Here's how the part is built. I have some questions about the finished solid (model axes, mm). A direction names the side the tool comes from. Round coordinates to 2 decimals unless told otherwise and drop trailing zeros. Loops run counter-clockwise (first coordinate to the right, second up) from the corner with the lowest first, then second, coordinate; pieces in that order, holes last. Notation, with made-up numbers: M 18,18 L 43,18 A24 cw 43,33 Z; hole C 13,54.5 d5. An arc over 180 degrees is marked long. Answer as a JSON object with one key per item and string values.
from build123d import *

# Parameters (mm, degrees)
F2_DEPTH  = 38.1
F3_W      = 25.4
F3_H      = 31.75
F4_DEPTH  = 25.4
F5_DEPTH  = 12.7
F7_D      = 12.7
F9_DEPTH  = 12.7
F10_DEPTH = 123
F11_R     = 5.08
F13_D     = 6.35
F15_D     = 6.35
F17_D     = 6.35


# Not quite as in the source:
# - an extrude ends at something that could not be found from the text; its depth is read off the source's solid


with BuildPart() as f2:
    # F0 (on Front) → F2 (new body)
    with BuildSketch(Plane.XZ):
        Polygon((-15.0914756011, 53.4695235106), (-53.1914756011, 53.4695235106), (-53.1914756011, 15.3695235106), (10.3085243989, 15.3695235106), (10.3085243989, 21.7195235106), (-15.0914756011, 21.7195235106), align=None)
    extrude(amount=F2_DEPTH)

    # F3 (on face) → F4 (cut)
    with BuildSketch(Plane.YZ.offset(-15.0914756011)):
        with Locations((-25.4, 37.5945235106)):
            Rectangle(F3_W, F3_H)
    extrude(amount=-F4_DEPTH, mode=Mode.SUBTRACT)

    # F5 (cut): a face of the model
    f5_faces = [f2.faces().sort_by_distance(p)[0] for p in [
        (-40.4914756011, -25.4, 37.5945235106),
    ]]
    extrude(f5_faces, amount=-F5_DEPTH, mode=Mode.SUBTRACT)

    # F7 (through all)
    with Locations(Plane.XZ.offset(12.7)):
        with Locations((-40.4914756011, 40.7695235106)):
            Hole(F7_D / 2)

    # F8 (on face) → F9 (cut)
    with BuildSketch(Plane.XZ.offset(12.7)):
        with BuildLine():
            ThreePointArc((-53.1914756011, 40.0317125094), (-40.0621213537, 52.2842661721), (-27.8065160195, 39.1577604642))
            Line((-27.8065160195, 39.1577604642), (-27.8065160195, 34.4195235106))
            ThreePointArc((-27.8065160195, 34.4195235106), (-24.0770508865, 25.4383560684), (-15.0914756011, 21.7195235106))
            Line((-15.0914756011, 21.7195235106), (-15.0914756011, 53.4695235106))
            Line((-15.0914756011, 53.4695235106), (-53.1914756011, 53.4695235106))
            Line((-53.1914756011, 53.4695235106), (-53.1914756011, 40.0317125094))
        make_face()
    extrude(amount=-F9_DEPTH, mode=Mode.SUBTRACT)

    # F1 (on face) → F10 (cut, through all)
    with BuildSketch(Plane.XZ):
        Polygon((-15.0914756011, 21.7195235106), (-15.0914756011, 53.4695235106), (-53.1914756011, 53.4695235106), (-53.1914756011, 15.3695235106), (10.3085243989, 15.3695235106), (10.3085243989, 21.7195235106), align=None)
    extrude(amount=-F10_DEPTH, mode=Mode.SUBTRACT)

    # F11
    f11_edges = [f2.edges().sort_by_distance(p)[0] for p in [
        (-53.191476, -38.1, 18.544524),
        (10.308524, -38.1, 18.544524),
    ]]
    fillet(f11_edges, radius=F11_R)

    # F13 (through all)
    with Locations(Plane.XY.offset(21.7195235106)):
        with Locations((-43.6664756011, -28.575)):
            Hole(F13_D / 2)

    # F15 (through all)
    with Locations(Plane.XY.offset(21.7195235106)):
        with Locations((0.7835243989, -9.525)):
            Hole(F15_D / 2)

    # F17 (through all)
    with Locations(Plane.XY.offset(21.7195235106)):
        with Locations((0.7835243989, -28.575)):
            Hole(F17_D / 2)


solid = f2.part
Item 1: On a 3-axis mill with a long thin cutter (end or side, diameter ignored), from which of +Z, -Z, +X, -X, +Y, -Y can I reach the whole of each face in a straight line? I mean faces 1 (the face through (-27.807, -6, 37)), 2 (the face through (8.86, -36.57, 18.59)). Say none if no direction works.
Resolved:
{"face 1": "+Z, +X, +Y, -Y", "face 2": "+Z, -Z, +X, -Y"}
Item 2: I want a section at B-B, the plane x = -36. Please give me the cut outline in (y, z).
Resolved:
{"outline": "M -38.1,15.37 L 0,15.37 L 0,36.28 L -12.7,36.28 L -12.7,21.72 L -38.1,21.72 Z; M -12.7,45.26 L 0,45.26 L 0,51.47 L -12.7,51.47 Z"}
Item 3: I want a section at C-C, the plane y = -30. Please give me the cut outline in (x, z), then the cut area to 3 significant figures.
Resolved:
{"outline": "M -53.19,15.37 L -46.5,15.37 L -46.5,21.72 L -53.19,21.72 Z; M -40.83,15.37 L -2.05,15.37 L -2.05,21.72 L -40.83,21.72 Z; M 3.62,15.37 L 10.31,15.37 L 10.31,21.72 L 3.62,21.72 Z", "area": "331 mm²"}
Item 4: I want a section at D-D, the plane x = 3. Please give me the cut outline in (y, z), then the cut area to 3 significant figures.
Resolved:
{"outline": "M -38.1,15.37 L -30.85,15.37 L -30.85,21.72 L -38.1,21.72 Z; M -26.3,15.37 L -11.8,15.37 L -11.8,21.72 L -26.3,21.72 Z; M -7.25,15.37 L 0,15.37 L 0,21.72 L -7.25,21.72 Z", "area": "184 mm²"}
Item 5: I'm going to push flat-ended pins straight in: pin 1 Ø6 at (x, y) = (-21, -8.5) entering from +Z; pin 2 Ø1 at (y, z) = (-9, 31) entering from +X; pin 3 Ø2.5 at (y, z) = (-3.5, 37.5) entering from +X. Where does each tip first touch, or does it pass through?
Resolved:
{"pin 1": "z = 25.36", "pin 2": "x = -27.18", "pin 3": "x = -27.81"}
Item 6: If we mould it in two halves opening along Y, with no side actions, what happens to faces 3 (the face through (1.472, -12.624, 18.5)), 4 (the face through (-36, 0, 30)), 5 (the face through (-38, -12.7, 33)), 6 (the face through (-21, -23, 21.72))? For each: pulls with the +Y half, pulls with the -Y half, needs draft (parallel to the pull), parting line crosses it, or undercut.
Resolved:
{"face 3": "undercut", "face 4": "pulls with the +Y half", "face 5": "pulls with the -Y half", "face 6": "needs draft"}
Item 7: Please list where these lines run through material, in increasing order: probe 1 along Y at (x, z) = (-37, 26); probe 2 along X at (y, z) = (-9.5, 19.5); probe 3 along Z at (x, y) = (-28, -23.5). Write a range as from..to.
Resolved:
{"probe 1": "-12.7..0", "probe 2": "-53.19..-2.39, 3.96..10.31", "probe 3": "15.37..21.72"}
